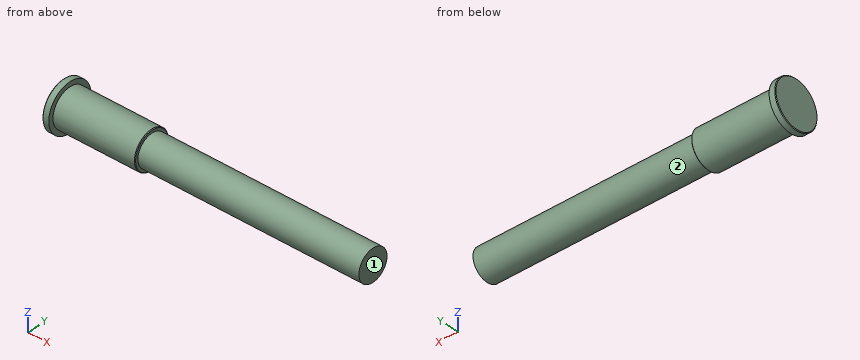
```python
from build123d import *

# Parameters (mm, degrees)
SKETCH1_R           = 7.5
BOSS_EXTRUDE1_DEPTH = 2
SKETCH2_R           = 6
BOSS_EXTRUDE2_DEPTH = 26
SKETCH3_R           = 5
BOSS_EXTRUDE3_DEPTH = 70
CHAMFER1_SIZE       = 0.2
SCALE1_SCALE        = 0.317565217


with BuildPart() as part:
    # Sketch1 → Boss-Extrude1 (new body)
    with BuildSketch(Plane(origin=(0, 0, 0), x_dir=(0, 0, -1), z_dir=(1, 0, 0))):
        Circle(SKETCH1_R)
    extrude(amount=BOSS_EXTRUDE1_DEPTH)

    # Sketch2 → Boss-Extrude2 (add)
    with BuildSketch(Plane(origin=(2, 0, 0), x_dir=(0, 0, -1), z_dir=(1, 0, 0))):
        with Locations(Location((0, 0, 0), (0, 0, 180))):
            Circle(SKETCH2_R)
    extrude(amount=BOSS_EXTRUDE2_DEPTH)

    # Sketch3 → Boss-Extrude3 (add)
    with BuildSketch(Plane(origin=(28, 0, 0), x_dir=(0, 0, -1), z_dir=(1, 0, 0))):
        Circle(SKETCH3_R)
    extrude(amount=BOSS_EXTRUDE3_DEPTH)

    # Chamfer1
    chamfer1_edges = [part.edges().sort_by_distance(p)[0] for p in [
        (0, 0, 7.5),
        (28, 0, -6),
    ]]
    chamfer(chamfer1_edges, length=CHAMFER1_SIZE)


with BuildPart() as part_1:
    # Scale1: scaled about (44.459396685, 0, 0)
    add(part.part.scale(SCALE1_SCALE).moved(Location((30.340638712, 0, 0))))


solid = part_1.part
```
CAD build for the part. Positions are in the model's coordinates, mm. Face numbers are marked on the shaded views. A direction names the side the tool comes from. Round coordinates to 2 decimals unless told otherwise and drop trailing zeros. Order: outer loops, then holes, each group sorted by start corner. A loop starts at its lowest first (then second) coordinate and runs counter-clockwise, first axis right, second up. Notation, with made-up numbers: (85, -39.75) - (124, -39.75) arc R19 ccw to (124, -20.75) - close; hole circle Ø4 at (-33, 7.25). An arc over 180 degrees is marked (long way). Use CSV: the item, a comma, the result in double quotes. Start each with the question number.
1) Tool access for the marked faces 1 and 2: list every direction of +Z, -Z, +X, -X, +Y, -Y with a clear straight run to the whole face (end or side of a thin tool).
2) Saw through at A-A (z = 0). List the corners of the cut face in (x, y), and give its area (3 significant figures).
3) Saw through at C-C (x = 49.5). List the corners of the cut face in (y, z), and give its area (3 significant figures).
4) Saw through at D-D (x = 33.5). List the corners of the cut face in (y, z), and give its area (3 significant figures).
5) Wall check: L1, parallel to X at y = 1.05, z = -1.25; L2, parallel to X at y = -1.5, z = -1.65; L3, parallel to Z at x = 37, y = 1.2. Give the ranges that are in metal, low to high. Write a range as [from, to].
Values follow:
1,face 1,"+Z, -Z, +X, +Y, -Y"
1,face 2,"+X"
2,outline,"(30.34, -2.32) - (30.4, -2.38) - (30.98, -2.38) - (30.98, -1.91) - (39.17, -1.91) - (39.23, -1.84) - (39.23, -1.59) - (61.46, -1.59) - (61.46, 1.59) - (39.23, 1.59) - (39.23, 1.84) - (39.17, 1.91) - (30.98, 1.91) - (30.98, 2.38) - (30.4, 2.38) - (30.34, 2.32) - close"
2,area,"105 mm2"
3,outline,"circle Ø3.18 at (0, 0)"
3,area,"7.92 mm2"
4,outline,"circle Ø3.81 at (0, 0)"
4,area,"11.4 mm2"
5,L1,"x = [30.34, 39.23]"
5,L2,"x = [30.34, 30.98]"
5,L3,"z = [-1.48, 1.48]"
